Can you work these out from the model? Positions are in its coordinate system, mm. Round coordinates to 2 decimals unless told otherwise and drop trailing zeros. Write each loop counter-clockwise with the first axis right and the second up, starting at its lowest first coordinate (ties: lowest second). Pieces come first, ordered by that corner, then holes. Notation, with made-up numbers: M 55,-20 L 61,-20 A29 cw 61,10 Z; hole C 27.5,-34 d5. An arc over 180 degrees is marked long. Answer in a Markdown table with one row per item. Add a question column.
(1) If I drill on probe 1 along X at (y, z) = (22, 0); probe 2 along Z at (x, y) = (22, 9); probe 3 along Y at (x, z) = (18.5, -9.5), over which ranges is the centre line in solid material (lowest first)?
(2) If we mould it in two halves opening along X, with no side actions, what happens to faces 1 (the face through (-32, 18, 7)), 2 (the face through (11.827, -18.727, -12.898)), 3 (the face through (32, 18, 7)), 4 (the face through (0, 29, -33))? For each: released by +X, released by -X, zero draft, split by the parting line, or undercut.
(3) I'm going to push a flat-ended pin straight in: pin 1 (12 mm diameter, centred on x = 18, z = 1.5, fed in from -Y). Where does the tip first touch, or does it pass through?
(4) Suppose I cut it at A-A, the plane z = 0. Write out the boundary of the cut face in (x, y).
(5) Suppose I cut it at B-B, the plane y = -19.5. Write out the boundary of the cut face in (x, z).
from build123d import *

# Parameters (mm, degrees)
SKETCH1_W           = 64
SKETCH1_H           = 70
BOSS_EXTRUDE1_DEPTH = 32
SKETCH2_R           = 17.5
CUT_EXTRUDE1_DEPTH  = 80.655508284
CIRPATTERN4_COUNT   = 4
CHAMFER1_SIZE       = 5
CHAMFER2_SIZE       = 1


with BuildPart() as part:
    # Sketch1 → Boss-Extrude1 (new, symmetric)
    with BuildSketch(Plane(origin=(0, 0, 0), x_dir=(1, 0, 0), z_dir=(0, 1, 0))):
        Rectangle(SKETCH1_W, SKETCH1_H)
    extrude(amount=BOSS_EXTRUDE1_DEPTH, both=True)

    # Sketch2 → Cut-Extrude1 (cut, through all)
    with BuildSketch(Plane(origin=(0, 32, 0), x_dir=(1, 0, 0), z_dir=(0, 1, 0))):
        with Locations(Location((0, 0, 0), (0, 0, 270))):
            Circle(SKETCH2_R)
    cut_extrude1 = extrude(amount=-CUT_EXTRUDE1_DEPTH, mode=Mode.SUBTRACT)

    # CirPattern4: Cut-Extrude1 ×4 about axis
    cirpattern4_axis = Axis((0, 0, 38.5), (0, 0, -1))
    for i in range(1, CIRPATTERN4_COUNT):
        add(cut_extrude1.rotate(cirpattern4_axis, i * 360 / CIRPATTERN4_COUNT), mode=Mode.SUBTRACT)

    # Chamfer1
    chamfer1_edges = [part.edges().sort_by_distance(p)[0] for p in [
        (-32, 32, 0),
        (0, 32, 35),
        (32, 32, 0),
        (0, -32, 35),
        (-32, -32, 0),
        (0, -32, -35),
        (32, -32, 0),
        (32, 0, 35),
        (-32, 0, 35),
        (-32, 0, -35),
        (32, 0, -35),
        (0, 32, -35),
    ]]
    chamfer(chamfer1_edges, length=CHAMFER1_SIZE)

    # Chamfer2
    chamfer2_edges = [part.edges().sort_by_distance(p)[0] for p in [
        (0, -32, -17.5),
        (0, 32, -17.5),
        (-32, 0, -17.5),
        (32, 0, -17.5),
    ]]
    chamfer(chamfer2_edges, length=CHAMFER2_SIZE)


solid = part.part
Calculated:
| question | item | result |
|---|---|---|
| 1 | probe 1 | -32 to -17.5, 17.5 to 32 |
| 1 | probe 2 | -35 to -15.01, 15.01 to 35 |
| 1 | probe 3 | -32 to -14.7, 14.7 to 32 |
| 2 | face 1 | released by -X |
| 2 | face 2 | undercut |
| 2 | face 3 | released by +X |
| 2 | face 4 | zero draft |
| 3 | pin 1 | y = -32 |
| 4 | outline | M -32,-27 L -27,-32 L -18.5,-32 L -17.5,-31 L -17.5,-17.5 L -31,-17.5 L -32,-18.5 Z; M -32,18.5 L -31,17.5 L -17.5,17.5 L -17.5,31 L -18.5,32 L -27,32 L -32,27 Z; M 17.5,-31 L 18.5,-32 L 27,-32 L 32,-27 L 32,-18.5 L 31,-17.5 L 17.5,-17.5 Z; M 17.5,17.5 L 31,17.5 L 32,18.5 L 32,27 L 27,32 L 18.5,32 L 17.5,31 Z |
| 5 | outline | M -32,-30 L -27,-35 L 27,-35 L 32,-30 L 32,30 L 27,35 L -27,35 L -32,30 Z; hole C 0,0 d35 |
